Can you work these out from the drawing? Everything is in mm from the part's minimum corner. Round coordinates to 2 decimals unless told otherwise and drop trailing zeros. Write each loop counter-clockwise with the first axis right and the second up, starting at its lowest first coordinate (ties: lowest second). Pieces come first, ordered by that corner, then holes. Notation, with made-up numbers: (-36, -32.5) -> (-10, -32.5) arc R21 ccw to (-10, -21.5) -> close; hole circle Ø3 at (21, -39). An arc over 180 degrees is marked (long way). Put each result on its own line as item: value. Start each with the question number.
1. Suppose I cut it at A-A (y = 4.25). Please give me the cut outline in (x, z), then the cut area to 3 significant figures.
2. For pin 1 (3 mm diameter, centred on y = 6.5, z = 22, fed in from -X); pin 2 (0.7 mm diameter, centred on y = 4, z = 24, fed in from -X); pin 3 (1.5 mm diameter, centred on x = 5.5, z = 7.5, fed in from +Y); pin 4 (3 mm diameter, centred on y = 5.5, z = 15.5, fed in from -X), each with a flat end and sliding along its axis, tell me the tip position at first contact or that it passes through.
3. We'd pull the mould along X, two halves only. Please class the marked faces 1, 2, 3 and 4: +X half, -X half, draft (parallel to the pull), parting line (faces both ways), or undercut.
4. Suppose I cut it at B-B (z = 15.75). Please give me the cut outline in (x, y), then the cut area to 3 significant figures.
5. I need wall thicknesses on probe 1 along Z at (x, y) = (1.5, 4.25); probe 2 along Z at (x, y) = (2.75, 4.5); probe 3 along X at (y, z) = (4.25, 7.25). Which ranges of each line are inside material? Lowest first, please. Write a range as from..to.
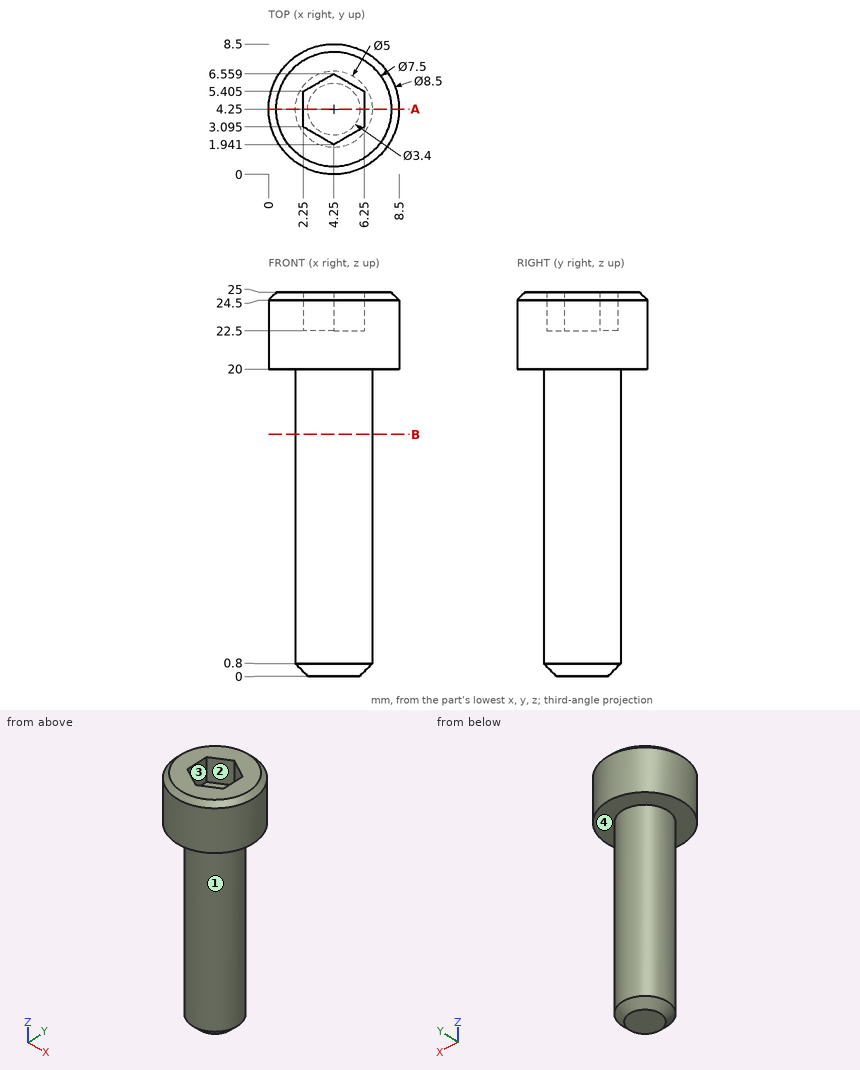
Verdict:
1. outline: (0, 20) -> (1.75, 20) -> (1.75, 0.8) -> (2.55, 0) -> (5.95, 0) -> (6.75, 0.8) -> (6.75, 20) -> (8.5, 20) -> (8.5, 24.5) -> (8, 25) -> (6.25, 25) -> (6.25, 22.5) -> (2.25, 22.5) -> (2.25, 25) -> (0.5, 25) -> (0, 24.5) -> close
1. area: 132 mm^2
2. pin 1: stops at x = 0.07
2. pin 2: stops at x = 0
2. pin 3: stops at y = 6.7
2. pin 4: stops at x = 1.75
3. face 1: parting line
3. face 2: undercut
3. face 3: undercut
3. face 4: draft
4. outline: circle Ø5 at (4.25, 4.25)
4. area: 19.6 mm^2
5. probe 1: z = 20..25
5. probe 2: z = 0..22.5
5. probe 3: x = 1.75..6.75
